```python
from build123d import *

# Parameters (mm, degrees)
F0_W     = 17.1407087726
F0_H     = 19.5990015107
F1_DEPTH = 35
F2_DEPTH = 25


with BuildPart() as f1:
    # F0 (on Top) → F1 (new body)
    with BuildSketch(Plane.XY):
        Rectangle(F0_W, F0_H)
        with BuildLine():
            ThreePointArc((-2.5, -6.5383484153), (-3.9686269666, 5.7662812973), (7, 0))
            ThreePointArc((7, 0), (5.7662812973, -3.9686269666), (2.5, -6.5383484153))
            Line((2.5, -6.5383484153), (2.5, -9.5))
            Line((2.5, -9.5), (0, -9.5))
            Line((0, -9.5), (-2.5, -9.5))
            Line((-2.5, -9.5), (-2.5, -6.5383484153))
        make_face(mode=Mode.SUBTRACT)
        with BuildLine():
            ThreePointArc((2.5, -6.5383484153), (5.7662812973, -3.9686269666), (7, 0))
            ThreePointArc((7, 0), (-3.9686269666, 5.7662812973), (-2.5, -6.5383484153))
            ThreePointArc((-2.5, -6.5383484153), (0, -7), (2.5, -6.5383484153))
        make_face()
        with BuildLine():
            ThreePointArc((2.5, -6.5383484153), (0, -7), (-2.5, -6.5383484153))
            Line((-2.5, -6.5383484153), (-2.5, -9.5))
            Line((-2.5, -9.5), (0, -9.5))
            Line((0, -9.5), (2.5, -9.5))
            Line((2.5, -9.5), (2.5, -6.5383484153))
        make_face()
    extrude(amount=F1_DEPTH)

    # F0 (on Top) → F2 (cut)
    with BuildSketch(Plane.XY):
        with BuildLine():
            ThreePointArc((2.5, -6.5383484153), (5.7662812973, -3.9686269666), (7, 0))
            ThreePointArc((7, 0), (-3.9686269666, 5.7662812973), (-2.5, -6.5383484153))
            ThreePointArc((-2.5, -6.5383484153), (0, -7), (2.5, -6.5383484153))
        make_face()
        with BuildLine():
            ThreePointArc((2.5, -6.5383484153), (0, -7), (-2.5, -6.5383484153))
            Line((-2.5, -6.5383484153), (-2.5, -9.5))
            Line((-2.5, -9.5), (0, -9.5))
            Line((0, -9.5), (2.5, -9.5))
            Line((2.5, -9.5), (2.5, -6.5383484153))
        make_face()
    extrude(amount=F2_DEPTH, mode=Mode.SUBTRACT)


solid = f1.part
```
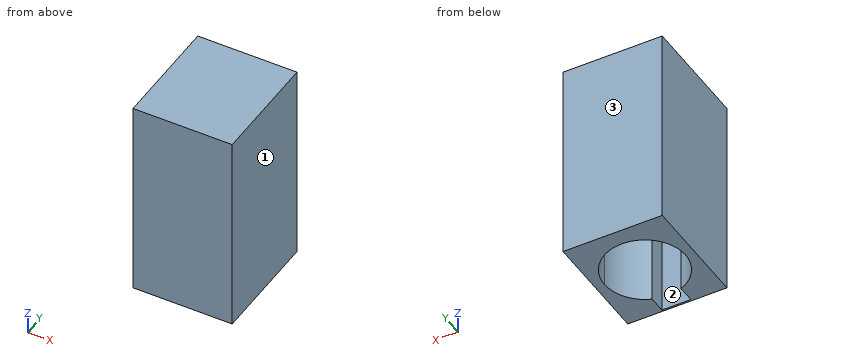
Part model, mm, in its own coordinate system. Face numbers are marked on the shaded views. Round coordinates to 2 decimals unless told otherwise and drop trailing zeros. Order: outer loops, then holes, each group sorted by start corner. A loop starts at its lowest first (then second) coordinate and runs counter-clockwise, first axis right, second up. Notation, with made-up numbers: M 31,32 L 69,32 A16 cw 69,56 Z; hole C 53,52 d4. An arc over 180 degrees is marked long. Put each result on its own line as item: value. Start each with the question number.
1. Drill centre lines: probe 1 along X at (y, z) = (-7.5, 3); probe 2 along Y at (x, z) = (0, 8); probe 3 along X at (y, z) = (0.25, 15.5). Where is each one in solid material? Low to high. Write a range as [from, to].
2. Two-plate mould, pull along X, no slides. Class the marked faces 1, 2 and 3: +X half, -X half, draft (parallel to the pull), parting line (faces both ways), or undercut.
3. Slice it at C-C on y = -4.5. List the corners of the cut face in (x, z).
4. Drop a flat-ended pin along its axis: pin 1 (3 mm diameter, centred on x = -3, y = 3, fed in from -Z). Give the stop position or say it passes through.
5. Slice it at B-B on x = 0. List the corners of the cut face in (y, z), then the cut area to 3 significant figures.
6. Slice it at A-A on z = 6. List the corners of the cut face in (x, y).
Findings:
1. probe 1: [-8.57, -2.5], [2.5, 8.57]
1. probe 2: [-9.8, -9.5], [7, 9.8]
1. probe 3: [-8.57, -7], [7, 8.57]
2. face 1: +X half
2. face 2: undercut
2. face 3: draft
3. outline: M -8.57,0 L -5.36,0 L -5.36,25 L 5.36,25 L 5.36,0 L 8.57,0 L 8.57,35 L -8.57,35 Z
4. pin 1: z = 25
5. outline: M -9.8,0 L -9.5,0 L -9.5,25 L 7,25 L 7,0 L 9.8,0 L 9.8,35 L -9.8,35 Z
5. area: 273 mm2
6. outline: M -8.57,-9.8 L 8.57,-9.8 L 8.57,9.8 L -8.57,9.8 Z; hole M -2.5,-9.5 L 2.5,-9.5 L 2.5,-6.54 A7 ccw long -2.5,-6.54 Z
